Here's how the part is built. I have some questions about the finished solid (model axes, mm). A direction names the side the tool comes from. Give positions to 0.01 mm unless a question says otherwise; leave off trailing zeros. Loops run counter-clockwise (first coordinate to the right, second up) from the corner with the lowest first, then second, coordinate; pieces in that order, holes last.
Q1. I'm going to push flat-ended pins straight in: P1, Ø1.2, axis at x = -1.5, z = -1.5, coming from the +Y side; P2, Ø1.2, axis at x = -2.5, z = -1.5, coming from the -Y side; P3, Ø1.5, axis at x = -2.5, y = -0.5, coming from the -Z side. Where does each tip first touch, or does it pass through?
Q2. Suppose I cut it at B-B (y = -1.75). List the corners of the cut face in (x, z) for me.
Q3. Suppose I cut it at A-A (x = 1.25). List the corners of the cut face in (y, z) for me.
Q4. Suppose I cut it at C-C (z = -0.45). List the corners of the cut face in (x, y) for me, and give its area (3 significant figures).
Q5. I need wall thicknesses on probe 1 along Y at (x, z) = (0, 0.8) (3 decimals); probe 2 along Z at (x, y) = (-6, -0.5); probe 3 along Y at (x, z) = (0.5, -0.05). Which ranges of each line are inside material? Lowest first, please.
Q6. Thinking about a two-plate mould opening in Y: for faces 3 (the face through (3, 0, 1)), 4 (the face through (-3, 0, 0)), 5 (the face through (-1.46, -6.59, 0.49)), which applies, pulls with the +Y half, pulls with the -Y half, needs draft (parallel to the pull), parting line crosses it, or undercut?
Q7. For faces 1 (the face through (4, 2, -2.5)), 2 (the face through (-2, -4.05, -1)), which set-ups out of +Z, -Z, +X, -X, +Y, -Y let a thin tool reach every point of the face, with its end or its side?
Q8. Suppose I cut it at D-D (x = -0.5). List the corners of the cut face in (y, z) for me, and give its area (3 significant figures).
```python
from build123d import *

# Parameters (mm, degrees)
F0_R     = 6.75
F0_R_2   = 2.725
F1_DEPTH = 1
F3_DEPTH = 2.5


with BuildPart() as f1:
    # F0 (on Top) → F1 (new body)
    with BuildSketch(Plane.XY):
        Circle(F0_R)
        Circle(F0_R_2, mode=Mode.SUBTRACT)
    extrude(amount=F1_DEPTH)

    # F2 (on face) → F3 (join)
    with BuildSketch(Plane(origin=(0, 0, 0), x_dir=(1, 0, 0), z_dir=(0, 0, -1))):
        with BuildLine():
            ThreePointArc((-4.0109225871, -4.05), (2.1940534694, -5.2608107145), (5.7, 0))
            ThreePointArc((5.7, 0), (2.1940534694, 5.2608107145), (-4.0109225871, 4.05))
            Line((-4.0109225871, 4.05), (0, 4.05))
            ThreePointArc((0, 4.05), (2.8637824638, 2.8637824638), (4.05, 0))
            ThreePointArc((4.05, 0), (2.8637824638, -2.8637824638), (0, -4.05))
            Line((0, -4.05), (-4.0109225871, -4.05))
        make_face()
    extrude(amount=F3_DEPTH)


solid = f1.part
```
Solutions:
1. P1: stops at y = 5.63
1. P2: stops at y = -5.37
1. P3: stops at z = 0
2. outline: (-6.52, 0) - (-2.09, 0) - (-2.09, 1) - (-6.52, 1) - close; (2.09, 0) - (3.65, 0) - (3.65, -2.5) - (5.42, -2.5) - (5.42, 0) - (6.52, 0) - (6.52, 1) - (2.09, 1) - close
3. outline: (-6.63, 0) - (-5.56, 0) - (-5.56, -2.5) - (-3.85, -2.5) - (-3.85, 0) - (-2.42, 0) - (-2.42, 1) - (-6.63, 1) - close; (2.42, 0) - (3.85, 0) - (3.85, -2.5) - (5.56, -2.5) - (5.56, 0) - (6.63, 0) - (6.63, 1) - (2.42, 1) - close
4. outline: (-4.01, -4.05) arc R5.7 ccw (long way) to (-4.01, 4.05) - (0, 4.05) arc R4.05 cw to (0, -4.05) - close
4. area: 34.4 mm2
5. probe 1: y = -6.75 to -2.725, 2.725 to 6.75
5. probe 2: z = 0 to 1
5. probe 3: y = -5.68 to -4.02, 4.02 to 5.68
6. face 3: needs draft
6. face 4: undercut
6. face 5: parting line crosses it
7. face 1: -Z, +X, -X, +Y, -Y
7. face 2: -Z, -X
8. outline: (-6.73, 0) - (-5.68, 0) - (-5.68, -2.5) - (-4.05, -2.5) - (-4.05, 0) - (-2.68, 0) - (-2.68, 1) - (-6.73, 1) - close; (2.68, 0) - (4.05, 0) - (4.05, -2.5) - (5.68, -2.5) - (5.68, 0) - (6.73, 0) - (6.73, 1) - (2.68, 1) - close
8. area: 16.2 mm2
